```python
from build123d import *

# Parameters (mm, degrees)
BOSS_EXTRUDE1_DEPTH = 0.31
SKETCH2_W           = 3
SKETCH2_H           = 0.31
BOSS_EXTRUDE2_DEPTH = 4
SKETCH3_R           = 0.65
CUT_EXTRUDE1_DEPTH  = 11
SKETCH4_W           = 3.66
SKETCH4_H           = 0.31
BOSS_EXTRUDE3_DEPTH = 4.82
SKETCH5_R           = 0.75
CUT_EXTRUDE2_DEPTH  = 4.82


with BuildPart() as part:
    # Sketch1 → Boss-Extrude1 (new body)
    with BuildSketch(Plane(origin=(0, 0, 0), x_dir=(1, 0, 0), z_dir=(0, 1, 0))):
        Polygon((0, 3.025), (0, -3.025), (3, -3.025), (3, -2.025), (4, -2.125), (14.38, -1.575), (14.38, -2), (18.04, -2), (18.04, 2), (14.38, 2), (14.38, 1.575), (4, 2.125), (3, 2.025), (3, 3.025), align=None)
    extrude(amount=BOSS_EXTRUDE1_DEPTH)

    # Sketch2 → Boss-Extrude2 (add)
    with BuildSketch(Plane(origin=(0, 0.31, 0), x_dir=(1, 0, 0), z_dir=(0, 1, 0))):
        with Locations((1.5, 2.87)):
            Rectangle(SKETCH2_W, SKETCH2_H)
        with Locations((1.5, -2.87)):
            Rectangle(SKETCH2_W, SKETCH2_H)
    extrude(amount=-BOSS_EXTRUDE2_DEPTH)

    # Sketch3 → Cut-Extrude1 (cut)
    with BuildSketch(Plane.XY.offset(3.025)):
        with Locations((1.5, -2.19)):
            Circle(SKETCH3_R)
        with BuildLine():
            ThreePointArc((3, -2.19), (2.560660172, -3.250660172), (1.5, -3.69))
            Line((1.5, -3.69), (3, -3.69))
            Line((3, -3.69), (3, -2.19))
        make_face()
        with BuildLine():
            ThreePointArc((1.5, -3.69), (0.439339828, -3.250660172), (0, -2.19))
            Line((0, -2.19), (0, -3.69))
            Line((0, -3.69), (1.5, -3.69))
        make_face()
    extrude(amount=-CUT_EXTRUDE1_DEPTH, mode=Mode.SUBTRACT)

    # Sketch4 → Boss-Extrude3 (add)
    with BuildSketch(Plane(origin=(0, 0.31, 0), x_dir=(1, 0, 0), z_dir=(0, 1, 0))):
        with Locations((16.21, 1.845)):
            Rectangle(SKETCH4_W, SKETCH4_H)
        with Locations((16.21, -1.845)):
            Rectangle(SKETCH4_W, SKETCH4_H)
    extrude(amount=BOSS_EXTRUDE3_DEPTH)

    # Sketch5 → Cut-Extrude2 (cut)
    with BuildSketch(Plane(origin=(0, 0, -2), x_dir=(-1, 0, 0), z_dir=(0, 0, -1))):
        with BuildLine():
            Line((-18.04, 5.13), (-18.04, 3.3))
            ThreePointArc((-18.04, 3.3), (-17.50400541, 4.59400541), (-16.21, 5.13))
            Line((-16.21, 5.13), (-18.04, 5.13))
        make_face()
        with BuildLine():
            Line((-14.38, 5.13), (-16.21, 5.13))
            ThreePointArc((-16.21, 5.13), (-14.91599459, 4.59400541), (-14.38, 3.3))
            Line((-14.38, 3.3), (-14.38, 5.13))
        make_face()
        with Locations((-16.21, 3.3)):
            Circle(SKETCH5_R)
    extrude(amount=-CUT_EXTRUDE2_DEPTH, mode=Mode.SUBTRACT)


solid = part.part
```
Could you check a few things on this model? Use its own coordinates, in mm. A direction names the side the tool comes from. Give positions to 0.01 mm unless a question says otherwise; leave off trailing zeros. Order: outer loops, then holes, each group sorted by start corner. A loop starts at its lowest first (then second) coordinate and runs counter-clockwise, first axis right, second up.
Q1. Suppose I cut it at D-D, the plane z = 1.25. Write out the boundary of the cut face in (x, y), and give its area (3 significant figures).
Q2. If I drill on line 1 along Y through (x, z) = (1.5, -2.85); line 2 along Y through (x, z) = (16.21, -1.75); line 3 along Z through (x, y) = (17.5, 1), over which ranges is the centre line in solid material (lowest first)?
Q3. For faces 1 (the flat face through (9, 0, 0)), 2 (the flat face through (16, 2, 2)), 3 (the flat face through (16, 2, 1.69)), which set-ups out of +Z, -Z, +X, -X, +Y, -Y let a thin tool reach every point of the face, with its end or its side?
Q4. Suppose I cut it at A-A, the plane y = 0.75. Write out the boundary of the cut face in (x, z).
Q5. We'd pull the mould along Z, two halves only. Please class faces 4 (the cylindrical face through (16.805, 2.844, 1.843)), 5 (the flat face through (16, 2, -2)), 6 (the flat face through (1, -1, 2.715)): +Z half, -Z half, draft (parallel to the pull), parting line (faces both ways), or undercut.
Q6. Suppose I cut it at C-C, the plane y = -1.75. Write out the boundary of the cut face in (x, z) (3 decimals), and give its area (3 significant figures).
Q7. Suppose I cut it at B-B, the plane x = 16.5. Write out the boundary of the cut face in (y, z).
Q8. I'm going to push flat-ended pins straight in: P1, Ø1.7, axis at x = 16.21, y = 3.3, coming from the +Z side; P2, Ø1, axis at x = 10.5, z = 1, coming from the +Y side; P3, Ø1.1, axis at x = 16, y = 1.5, coming from the -Z side. Where does each tip first touch, or does it pass through?
Solution:
1. outline: (0, 0) - (18.04, 0) - (18.04, 0.31) - (0, 0.31) - close
1. area: 5.59 mm2
2. line 1: y = -3.69 to -2.84, -1.54 to 0.31
2. line 2: y = 0 to 2.55, 4.05 to 5.13
2. line 3: z = -2 to -1.69, 1.69 to 2
3. face 1: +X, -X, -Y
3. face 2: +Z, +X, +Y, -Y
3. face 3: +X, -X, +Y
4. outline: (14.38, -2) - (18.04, -2) - (18.04, -1.69) - (14.38, -1.69) - close; (14.38, 1.69) - (18.04, 1.69) - (18.04, 2) - (14.38, 2) - close
5. face 4: draft
5. face 5: -Z half
5. face 6: undercut
6. outline: (0, -3.025) - (1.022, -3.025) - (1.022, -2.715) - (0, -2.715) - close; (0, 2.715) - (1.022, 2.715) - (1.022, 3.025) - (0, 3.025) - close; (1.978, -3.025) - (3, -3.025) - (3, -2.715) - (1.978, -2.715) - close; (1.978, 2.715) - (3, 2.715) - (3, 3.025) - (1.978, 3.025) - close
6. area: 1.27 mm2
7. outline: (0, -2) - (2.61, -2) - (2.61, -1.69) - (0.31, -1.69) - (0.31, 1.69) - (2.61, 1.69) - (2.61, 2) - (0, 2) - close; (3.99, -2) - (5.11, -2) - (5.11, -1.69) - (3.99, -1.69) - close; (3.99, 1.69) - (5.11, 1.69) - (5.11, 2) - (3.99, 2) - close
8. P1: stops at z = 2
8. P2: stops at y = 0.31
8. P3: stops at z = -2
